Geometry check sheet. Reference: the model listing, model coordinates, mm. A direction names the side the tool comes from. Coordinates: 2 decimals unless noted, no trailing zeros. Write each loop counter-clockwise with the first axis right and the second up, starting at its lowest first coordinate (ties: lowest second). Pieces come first, ordered by that corner, then holes. Notation, with made-up numbers: M -21,79.5 L -1,79.5 A25 cw -1,95.5 Z; hole C 59.25,-28.75 d6. An arc over 180 degrees is marked long. Put each result on its own line as item: value. Start each with the question number.
1) Cross-section at A-A on y = 0. Record the cut outline in (x, z) (3 decimals).
2) Cross-section at D-D on y = -18. Record the cut outline in (x, z) (3 decimals), plus the area to 3 significant figures.
3) Cross-section at B-B on z = 3.5. Record the cut outline in (x, y) (3 decimals).
4) Gauge pin test, flat ends, axial feed: pin 1 (1.9 mm diameter, centred on x = 15.5, z = 3.5, fed in from -Y); pin 2 (21 mm diameter, centred on x = 0.5, y = 7.5, fed in from +Z). Record the tip position at first contact, or that the pin passes through.
5) Scan lines: line 1 along X through (y, z) = (-10.5, 3.5) (3 decimals); line 2 along X through (y, z) = (-8, 0.5); line 3 along Y through (x, z) = (-1, 2.75). Record each from-to range of solid material in increasing order.
6) Mould release check, pull along X, two halves, no side actions. Record for faces 4 (the flat face through (0, -23, 3)), 5 (the flat face through (18, 0, 3)), 6 (the flat face through (6, 0, 1)): released by +X, released by -X, zero draft, split by the parting line, or undercut.
7) Set-up check for faces 1 (the flat face through (0, -21, 4)), 2 (the cylindrical face through (17.038, 0.322, 3.841)), 3 (the cylindrical face through (5, -18.5, 1)): record each of +Z, -Z, +X, -X, +Y, -Y from which the full face is reachable in a straight line by a thin tool's end or side.
8) Cross-section at C-C on x = -5. Record the cut outline in (y, z), plus the area to 3 significant figures.
from build123d import *

# Parameters (mm, degrees)
SKETCH1_W           = 36
SKETCH1_H           = 46
BOSS_EXTRUDE1_DEPTH = 2
SKETCH2_W           = 36
SKETCH2_H           = 46
SKETCH2_W_2         = 26
SKETCH2_H_2         = 42
BOSS_EXTRUDE2_DEPTH = 5
SKETCH3_R           = 1.575
CUT_EXTRUDE1_DEPTH  = 50.889878733
CUT_EXTRUDE2_DEPTH  = 2


with BuildPart() as part:
    # Sketch1 → Boss-Extrude1 (new body)
    with BuildSketch(Plane.XY):
        Rectangle(SKETCH1_W, SKETCH1_H)
    extrude(amount=BOSS_EXTRUDE1_DEPTH)

    # Sketch2 → Boss-Extrude2 (add)
    with BuildSketch(Plane.XY.offset(2)):
        Rectangle(SKETCH2_W, SKETCH2_H)
        Rectangle(SKETCH2_W_2, SKETCH2_H_2, mode=Mode.SUBTRACT)
    extrude(amount=BOSS_EXTRUDE2_DEPTH)

    # Sketch3 → Cut-Extrude1 (cut, through all)
    with BuildSketch(Plane(origin=(0, 23, 0), x_dir=(1, 0, 0), z_dir=(0, 1, 0))):
        with Locations(Location((-15.5, -3.5, 0), (0, 0, 270))):
            Circle(SKETCH3_R)
        with Locations(Location((15.5, -3.5, 0), (0, 0, 90))):
            Circle(SKETCH3_R)
    extrude(amount=-CUT_EXTRUDE1_DEPTH, mode=Mode.SUBTRACT)

    # Sketch4 → Cut-Extrude2 (cut)
    with BuildSketch(Plane(origin=(0, 0, 0), x_dir=(-1, 0, 0), z_dir=(0, 0, -1))):
        with BuildLine():
            Line((-4, 17.5), (-4, -17.5))
            ThreePointArc((-4, -17.5), (-5, -18.5), (-6, -17.5))
            Line((-6, -17.5), (-6, 17.5))
            ThreePointArc((-6, 17.5), (-5, 18.5), (-4, 17.5))
        make_face()
        with BuildLine():
            Line((4, 17.5), (4, -17.5))
            ThreePointArc((4, -17.5), (5, -18.5), (6, -17.5))
            Line((6, -17.5), (6, 17.5))
            ThreePointArc((6, 17.5), (5, 18.5), (4, 17.5))
        make_face()
    extrude(amount=-CUT_EXTRUDE2_DEPTH, mode=Mode.SUBTRACT)


solid = part.part
Answer key:
1. outline: M -18,0 L -6,0 L -6,2 L -13,2 L -13,7 L -18,7 Z; M -4,0 L 4,0 L 4,2 L -4,2 Z; M 6,0 L 18,0 L 18,7 L 13,7 L 13,2 L 6,2 Z; hole C -15.5,3.5 d3.15; hole C 15.5,3.5 d3.15
2. outline: M -18,0 L -5.866,0 L -5.866,2 L -13,2 L -13,7 L -18,7 Z; M -4.134,0 L 4.134,0 L 4.134,2 L -4.134,2 Z; M 5.866,0 L 18,0 L 18,7 L 13,7 L 13,2 L 5.866,2 Z; hole C -15.5,3.5 d3.15; hole C 15.5,3.5 d3.15
2. area: 99.5 mm²
3. outline: M -18,-23 L -17.075,-23 L -17.075,23 L -18,23 Z; M -13.925,-23 L 13.925,-23 L 13.925,23 L -13.925,23 Z; M 17.075,-23 L 18,-23 L 18,23 L 17.075,23 Z; hole M -13,-21 L 13,-21 L 13,21 L -13,21 Z
4. pin 1: passes through
4. pin 2: stops at z = 2
5. line 1: x = -18 to -17.075, -13.925 to -13, 13 to 13.925, 17.075 to 18
5. line 2: x = -18 to -6, -4 to 4, 6 to 18
5. line 3: y = -23 to -21, 21 to 23
6. face 4: zero draft
6. face 5: released by +X
6. face 6: undercut
7. face 1: +Z
7. face 2: +Y, -Y
7. face 3: +Z, -Z
8. outline: M -23,0 L -18.5,0 L -18.5,2 L -21,2 L -21,7 L -23,7 Z; M 18.5,0 L 23,0 L 23,7 L 21,7 L 21,2 L 18.5,2 Z
8. area: 38.0 mm²
